Here's how the part is built. I have some questions about the finished solid (model axes, mm). A direction names the side the tool comes from. Give positions to 0.01 mm unless a question says otherwise; leave off trailing zeros. Write each loop counter-clockwise with the first axis right and the second up, starting at its lowest first coordinate (ties: lowest second). Pieces come first, ordered by that corner, then holes. Notation, with made-up numbers: (40, -36) - (52, -36) arc R31 ccw to (52, -8) - close; hole circle Ø2 at (-22, 2.5). An arc over 180 degrees is marked (long way). Use a Markdown table: item, result.
```python
from build123d import *

# Parameters (mm, degrees)
EXTRUDE_1_DEPTH          = 4
EXTRUDE_2_DEPTH          = 4
SKETCH_3_R               = 5
CUT_EXTRUDE_1_DEPTH      = 4
SKETCH_6_W               = 25
SKETCH_6_H               = 6
CUT_EXTRUDE_4_DEPTH      = 1
CUT_EXTRUDE_4_DEPTH_BACK = 5
SKETCH_7_R               = 2.025
CUT_EXTRUDE_5_DEPTH      = 1
CUT_EXTRUDE_5_DEPTH_BACK = 5
SKETCH_9_R               = 5
EXTRUDE_3_DEPTH          = 4
SKETCH_12_R              = 2.025
CUT_EXTRUDE_8_DEPTH      = 1
CUT_EXTRUDE_8_DEPTH_BACK = 5
EXTRUDE_4_DEPTH          = 4
FILLET_1_R               = 3


with BuildPart() as part:
    # 草图1 → 凸台-拉伸1 (new body)
    with BuildSketch(Plane.XY):
        Polygon((-35, 0), (0, 0), (0, -30), (25, -30), (25, 20), (-35, 20), align=None)
    extrude(amount=EXTRUDE_1_DEPTH)

    # 草图2 → 凸台-拉伸2 (add)
    with BuildSketch(Plane(origin=(0, 0, 0), x_dir=(-1, 0, 0), z_dir=(0, 0, -1))):
        with BuildLine():
            Line((-15.347247215, 38.473341973), (-25, 20))
            Line((-25, 20), (7.6, 20))
            Line((7.6, 20), (-2.052752785, 38.473341973))
            ThreePointArc((-2.052752785, 38.473341973), (-8.7, 42.5), (-15.347247215, 38.473341973))
        make_face()
    extrude(amount=-EXTRUDE_2_DEPTH)

    # 草图3 → 切除-拉伸1 (cut)
    with BuildSketch(Plane(origin=(0, 0, 0), x_dir=(-1, 0, 0), z_dir=(0, 0, -1))):
        with Locations((-8.7, 35)):
            Circle(SKETCH_3_R)
    extrude(amount=-CUT_EXTRUDE_1_DEPTH, mode=Mode.SUBTRACT)

    # 草图6 → 切除-拉伸4 (cut, two sides)
    with BuildSketch(Plane(origin=(0, 0, 0), x_dir=(-1, 0, 0), z_dir=(0, 0, -1))) as cut_extrude_4_sk:
        with Locations((-12.5, -27)):
            Rectangle(SKETCH_6_W, SKETCH_6_H)
    extrude(amount=CUT_EXTRUDE_4_DEPTH, mode=Mode.SUBTRACT)
    extrude(cut_extrude_4_sk.sketch, amount=-CUT_EXTRUDE_4_DEPTH_BACK, mode=Mode.SUBTRACT)

    # 草图7 → 切除-拉伸5 (cut, two sides)
    with BuildSketch(Plane(origin=(0, 0, 0), x_dir=(-1, 0, 0), z_dir=(0, 0, -1))) as cut_extrude_5_sk:
        with Locations((-12.5, -8)):
            Circle(SKETCH_7_R)
        with Locations((-12.5, -18)):
            Circle(SKETCH_7_R)
    extrude(amount=CUT_EXTRUDE_5_DEPTH, mode=Mode.SUBTRACT)
    extrude(cut_extrude_5_sk.sketch, amount=-CUT_EXTRUDE_5_DEPTH_BACK, mode=Mode.SUBTRACT)

    # 草图9 → 凸台-拉伸3 (add)
    with BuildSketch(Plane(origin=(0, 0, 0), x_dir=(-1, 0, 0), z_dir=(0, 0, -1))):
        with BuildLine():
            Line((-20.878399595, 37.817194226), (-25, 20))
            Line((-25, 20), (7.6, 20))
            Line((7.6, 20), (3.478399595, 37.817194226))
            ThreePointArc((3.478399595, 37.817194226), (-8.7, 47.5), (-20.878399595, 37.817194226))
        make_face()
        with Locations((-8.7, 35)):
            Circle(SKETCH_9_R, mode=Mode.SUBTRACT)
    extrude(amount=-EXTRUDE_3_DEPTH)

    # 草图12 → 切除-拉伸8 (cut, two sides)
    with BuildSketch(Plane(origin=(0, 0, 0), x_dir=(-1, 0, 0), z_dir=(0, 0, -1))) as cut_extrude_8_sk:
        with Locations((-15, 10)):
            Circle(SKETCH_12_R)
        with Locations((5, 10)):
            Circle(SKETCH_12_R)
        with Locations((25, 10)):
            Circle(SKETCH_12_R)
    extrude(amount=CUT_EXTRUDE_8_DEPTH, mode=Mode.SUBTRACT)
    extrude(cut_extrude_8_sk.sketch, amount=-CUT_EXTRUDE_8_DEPTH_BACK, mode=Mode.SUBTRACT)

    # 草图13 → 凸台-拉伸4 (add)
    with BuildSketch(Plane(origin=(0, 0, 0), x_dir=(-1, 0, 0), z_dir=(0, 0, -1))):
        Polygon((0, -6), (6, 0), (0, 0), align=None)
    extrude(amount=-EXTRUDE_4_DEPTH)

    # 圆角1
    fillet_1_edges = [part.edges().sort_by_distance(p)[0] for p in [
        (-6, 0, 2),
        (0, -6, 2),
        (-35, 20, 2),
        (25, 20, 2),
        (-35, 0, 2),
        (-7.6, 20, 2),
        (25, -24, 2),
        (0, -24, 2),
    ]]
    fillet(fillet_1_edges, radius=FILLET_1_R)


solid = part.part
```
Item 1: I need wall thicknesses on line 1 along Y through (x, z) = (12.5, 2.75) (3 decimals); line 2 along Y through (x, z) = (12, 0.7); line 3 along Y through (x, z) = (8, 3.8). Which ranges of each line are inside material? Lowest first, please. Write a range as [from, to].
Values:
| item | result |
|---|---|
| line 1 | y = [-24, -20.025], [-15.975, -10.025], [-5.975, 31.75], [38.25, 46.908] |
| line 2 | y = [-24, -19.96], [-16.04, -9.96], [-6.04, 31.24], [38.76, 47.06] |
| line 3 | y = [-24, 30.05], [39.95, 47.48] |
Item 2: For faces 1 (the flat face through (0, -14, 2)), 2 (the flat face through (-35, 10, 2)), 3 (the flat face through (-21, 20, 2)), which set-ups out of +Z, -Z, +X, -X, +Y, -Y let a thin tool reach every point of the face, with its end or its side?
Values:
| item | result |
|---|---|
| face 1 | +Z, -Z, -X, -Y |
| face 2 | +Z, -Z, -X, +Y, -Y |
| face 3 | +Z, -Z, -X, +Y |
Item 3: Thinking about a two-plate mould opening in Y: for faces 4 (the cylindrical face through (-23.39, 8.77, 1.97)), 5 (the cylindrical face through (-8.096, 20.669, 2.028)), 6 (the flat face through (-20, 0, 2)), which applies, +Y half, -Y half, draft (parallel to the pull), parting line (faces both ways), or undercut?
Values:
| item | result |
|---|---|
| face 4 | undercut |
| face 5 | +Y half |
| face 6 | -Y half |
Item 4: If we section it at D-D, the plane y = 41.5: Write out the boundary of the cut face in (x, z), plus the area to 3 significant figures.
Values:
| item | result |
|---|---|
| outline | (-1.98, 0) - (19.38, 0) - (19.38, 4) - (-1.98, 4) - close |
| area | 85.4 mm2 |
Item 5: If we section it at C-C, the plane z = 1.65: Write out the boundary of the cut face in (x, y) (3 decimals).
Values:
| item | result |
|---|---|
| outline | (-35, 3) arc R3 ccw to (-32, 0) - (-7.243, 0) arc R3 cw to (-5.121, -0.879) - (-0.879, -5.121) arc R3 cw to (0, -7.243) - (0, -21) arc R3 ccw to (3, -24) - (22, -24) arc R3 ccw to (25, -21) - (25, 19.658) arc R3 ccw to (24.923, 20.334) - (20.878, 37.817) arc R12.5 ccw to (-3.478, 37.817) - (-7.062, 22.324) arc R3 cw to (-9.985, 20) - (-32, 20) arc R3 ccw to (-35, 17) - close; hole circle Ø4.05 at (-25, 10); hole circle Ø4.05 at (-5, 10); hole circle Ø10 at (8.7, 35); hole circle Ø4.05 at (12.5, -18); hole circle Ø4.05 at (12.5, -8); hole circle Ø4.05 at (15, 10) |
Item 6: If we section it at A-A, the plane x = 8.7: Write out the boundary of the cut face in (y, z).
Values:
| item | result |
|---|---|
| outline | (-24, 0) - (30, 0) - (30, 4) - (-24, 4) - close; (40, 0) - (47.5, 0) - (47.5, 4) - (40, 4) - close |
Item 7: If we section it at B-B, the plane y = -8: Write out the boundary of the cut face in (x, z) (3 decimals), plus the area to 3 significant figures.
Values:
| item | result |
|---|---|
| outline | (0, 0) - (10.475, 0) - (10.475, 4) - (0, 4) - close; (14.525, 0) - (25, 0) - (25, 4) - (14.525, 4) - close |
| area | 83.8 mm2 |
Item 8: Will these pins go through, and if not, where does the flat tip stop? pin 1 Ø1 at (x, z) = (-8.5, 3) entering from -Y; pin 2 Ø2.5 at (x, y) = (12.5, -18) entering from +Z.
Values:
| item | result |
|---|---|
| pin 1 | stops at y = 0 |
| pin 2 | passes through |
